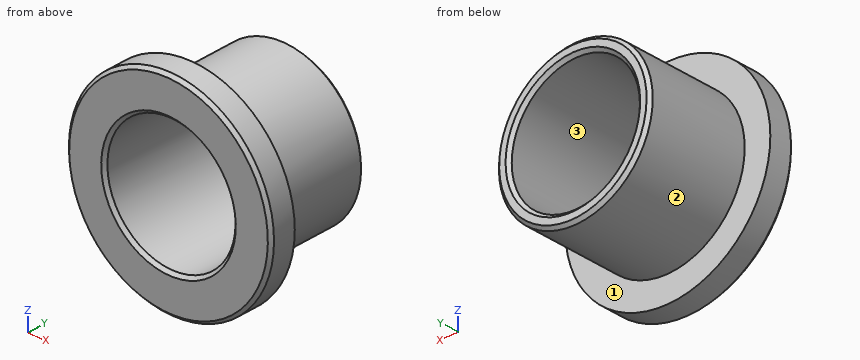
from build123d import *

# Parameters (mm, degrees)
SKETCH_1_R      = 8
SKETCH_1_R_2    = 5
EXTRUDE_1_DEPTH = 2
SKETCH_2_R      = 6
SKETCH_2_R_2    = 5
EXTRUDE_2_DEPTH = 8
CHAMFER_1_SIZE  = 0.25


with BuildPart() as part:
    # 草图1 → 凸台-拉伸1 (new body)
    with BuildSketch(Plane(origin=(0, 0, 0), x_dir=(1, 0, 0), z_dir=(0, 1, 0))):
        with Locations(Location((0, 0, 0), (0, 0, 270))):
            Circle(SKETCH_1_R)
        with Locations(Location((0, 0, 0), (0, 0, 270))):
            Circle(SKETCH_1_R_2, mode=Mode.SUBTRACT)
    extrude(amount=EXTRUDE_1_DEPTH)

    # 草图2 → 凸台-拉伸2 (add)
    with BuildSketch(Plane(origin=(0, 2, 0), x_dir=(1, 0, 0), z_dir=(0, 1, 0))):
        with Locations(Location((0, 0, 0), (0, 0, 270))):
            Circle(SKETCH_2_R)
        with Locations(Location((0, 0, 0), (0, 0, 270))):
            Circle(SKETCH_2_R_2, mode=Mode.SUBTRACT)
    extrude(amount=EXTRUDE_2_DEPTH)

    # 倒角1
    chamfer_1_edges = [part.edges().sort_by_distance(p)[0] for p in [
        (0, 10, -6),
        (0, 10, -5),
        (0, 0, -8),
        (0, 0, -5),
    ]]
    chamfer(chamfer_1_edges, length=CHAMFER_1_SIZE)


solid = part.part
The model under review builds one solid part; all positions refer to its coordinate system, in mm. Face numbers are marked on the shaded views. Give positions to 0.01 mm unless a question says otherwise; leave off trailing zeros. Order: outer loops, then holes, each group sorted by start corner. A loop starts at its lowest first (then second) coordinate and runs counter-clockwise, first axis right, second up. Notation, with made-up numbers: M 36,-19.75 L 82,-19.75 A32 ccw 82,8.25 Z; hole C -30,-6 d5. An arc over 180 degrees is marked long. One line per question, with ' | ' between items. Start each with the question number.
1) Consider section C-C, the plane y = 8. Give the boundary of the cut face in (x, z).
2) Mouldability with a two-part tool opening along X and no side actions: class the marked faces 1, 2 and 3 as pulls with the +X half, pulls with the -X half, needs draft (parallel to the pull), parting line crosses it, or undercut.
3) Wall thickness on L1, parallel to X at y = 3.5, z = 0; L2, parallel to Y at x = 3.75, z = -5.5; L3, parallel to Z at x = -1, y = 7.75: over which ranges is each line inside the solid? List them lowest first. Write a range as from..to.
4) Consider section A-A, the plane x = 0. Give the boundary of the cut face in (y, z).
5) Consider section B-B, the plane y = 1.5. Give the boundary of the cut face in (x, z), then the cut area to 3 significant figures.
6) Clearance check with flat-ended pins moving along their axes: P1, Ø1.5, axis at y = 2.5, z = -6, coming from the +X side; P2, Ø1.5, axis at x = 3, y = 2.5, coming from the +Z side; P3, Ø1.5, axis at x = -3, z = 2, coming from the -Y side; P4, Ø3, axis at x = 4.5, y = 6, coming from the -Z side. State where each tip first meets the part, or that it passes through.
Found:
1) outline: C 0,0 d12; hole C 0,0 d10
2) face 1: needs draft | face 2: parting line crosses it | face 3: undercut
3) L1: x = -6..-5, 5..6 | L2: y = 0..2 | L3: z = -5.92..-4.9, 4.9..5.92
4) outline: M 0,-7.75 L 0.25,-8 L 2,-8 L 2,-6 L 9.75,-6 L 10,-5.75 L 10,-5.25 L 9.75,-5 L 0.25,-5 L 0,-5.25 Z; M 0,5.25 L 0.25,5 L 9.75,5 L 10,5.25 L 10,5.75 L 9.75,6 L 2,6 L 2,8 L 0.25,8 L 0,7.75 Z
5) outline: C 0,0 d16; hole C 0,0 d10 | area: 123 mm²
6) P1: stops at x = 5.86 | P2: stops at z = 7.62 | P3: passes through | P4: stops at z = -5.2
